The listing builds one solid part. Answer for the finished solid, in the listing's coordinates (mm). Face numbers are marked on the shaded views. A direction names the side the tool comes from. Give positions to 0.01 mm unless a question says otherwise; leave off trailing zeros. Write each loop counter-clockwise with the first axis right and the second up, starting at its lowest first coordinate (ties: lowest second). Pieces come first, ordered by that corner, then holes. Notation, with made-up numbers: (4.25, 28.25) - (48.25, 28.25) arc R21 cw to (48.25, 62.25) - close; hole circle Ø3 at (-23, 29.25). An arc over 180 degrees is marked (long way). Return JSON: item names as keys, results as strings.
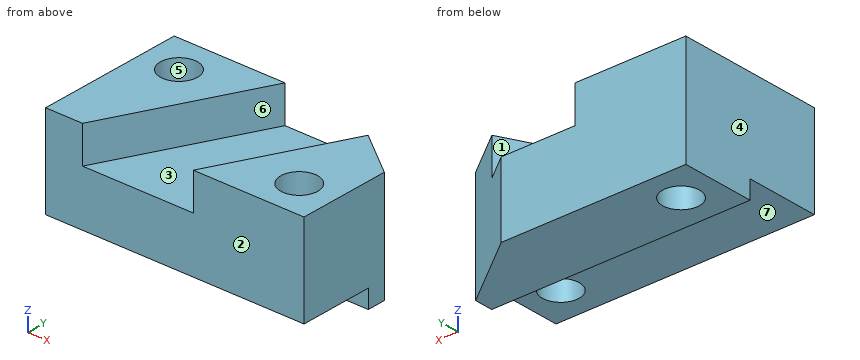
from build123d import *

# Parameters (mm, degrees)
SKETCH1_W               = 70
SKETCH1_H               = 30
BOSS_EXTRUDE1_DEPTH     = 40
CUT_EXTRUDE1_DEPTH      = 10
CUT_EXTRUDE2_DEPTH      = 1
CUT_EXTRUDE2_DEPTH_BACK = 31
SKETCH4_W               = 5
SKETCH4_H               = 20
CUT_EXTRUDE3_DEPTH      = 71
SKETCH5_R               = 5
CUT_EXTRUDE4_DEPTH      = 31
SKETCH6_R               = 5
CUT_EXTRUDE5_DEPTH      = 31


with BuildPart() as part:
    # Sketch1 → Boss-Extrude1 (new body)
    with BuildSketch(Plane(origin=(0, 0, 0), x_dir=(1, 0, 0), z_dir=(0, 1, 0))):
        with Locations((35, 15)):
            Rectangle(SKETCH1_W, SKETCH1_H)
    extrude(amount=BOSS_EXTRUDE1_DEPTH)

    # Sketch2 → Cut-Extrude1 (cut)
    with BuildSketch(Plane.XY):
        Polygon((30, 40), (10, 0), (40, 0), (60, 40), align=None)
    extrude(amount=-CUT_EXTRUDE1_DEPTH, mode=Mode.SUBTRACT)

    # Sketch3 → Cut-Extrude2 (cut, two sides)
    with BuildSketch(Plane(origin=(0, 0, -30), x_dir=(-1, 0, 0), z_dir=(0, 0, -1))) as cut_extrude2_sk:
        Polygon((-70, 40), (-70, 25), (-50, 40), align=None)
    extrude(amount=CUT_EXTRUDE2_DEPTH, mode=Mode.SUBTRACT)
    extrude(cut_extrude2_sk.sketch, amount=-CUT_EXTRUDE2_DEPTH_BACK, mode=Mode.SUBTRACT)

    # Sketch4 → Cut-Extrude3 (cut, through all)
    with BuildSketch(Plane(origin=(70, 0, 0), x_dir=(0, 0, -1), z_dir=(1, 0, 0))):
        with Locations((27.5, 10)):
            Rectangle(SKETCH4_W, SKETCH4_H)
    extrude(amount=-CUT_EXTRUDE3_DEPTH, mode=Mode.SUBTRACT)

    # Sketch5 → Cut-Extrude4 (cut, through all)
    with BuildSketch(Plane.XY):
        with Locations((60, 10)):
            Circle(SKETCH5_R)
    extrude(amount=-CUT_EXTRUDE4_DEPTH, mode=Mode.SUBTRACT)

    # Sketch6 → Cut-Extrude5 (cut, through all)
    with BuildSketch(Plane.XY):
        with Locations((10, 30)):
            Circle(SKETCH6_R)
    extrude(amount=-CUT_EXTRUDE5_DEPTH, mode=Mode.SUBTRACT)


solid = part.part
Item 1: Flat-ended cylindrical pins translate along their axes: P1, Ø8, axis at x = 51.5, y = 11, coming from the -Z side; P2, Ø2.5, axis at x = 32, z = -28, coming from the -Y side. Find the tip coordinate at first contact, or state that the pin passes through.
Answer below:
{"P1": "stops at z = -25", "P2": "stops at y = 20"}
Item 2: A cutting plane is placed at C-C on z = -22.5. Determine the outline of the cut face in (x, y).
Answer below:
{"outline": "(0, 0) - (70, 0) - (70, 25) - (50, 40) - (0, 40) - close; hole circle Ø10 at (10, 30); hole circle Ø10 at (60, 10)"}
Item 3: A cutting plane is placed at D-D on x = 18.5. Determine the outline of the cut face in (y, z).
Answer below:
{"outline": "(0, -25) - (20, -25) - (20, -30) - (40, -30) - (40, 0) - (17, 0) - (17, -10) - (0, -10) - close"}
Item 4: Consider L1, parallel to X at y = 7, z = -2.5; L2, parallel to X at y = 6, z = -1.25; L3, parallel to Y at x = 44, z = -26.75. Determine where each line is inside the solid, lowest interval first.
Answer below:
{"L1": "x = 0 to 13.5, 43.5 to 56, 64 to 70", "L2": "x = 0 to 13, 43 to 57, 63 to 70", "L3": "y = 20 to 40"}
Item 5: For the marked faces 1, 2 and 3, determine the directions among +Z, -Z, +X, -X, +Y, -Y from which every point of the face is accessible in a straight line to the end or side of a thin tool.
Answer below:
{"face 1": "+Z, +Y", "face 2": "+Z, -Z, +X, -X, -Y", "face 3": "+Z"}
Item 6: The mould has two halves that part along X. Classify the marked faces 4, 5, 6 and 7: +X half, -X half, draft (parallel to the pull), parting line (faces both ways), or undercut.
Answer below:
{"face 4": "-X half", "face 5": "undercut", "face 6": "undercut", "face 7": "draft"}
Item 7: A cutting plane is placed at B-B on x = 56. Determine the outline of the cut face in (y, z).
Answer below:
{"outline": "(0, -25) - (7, -25) - (7, 0) - (0, 0) - close; (13, -25) - (20, -25) - (20, -30) - (35.5, -30) - (35.5, -10) - (32, -10) - (32, 0) - (13, 0) - close"}
Item 8: A cutting plane is placed at A-A on y = 10. Determine the outline of the cut face in (x, z), then the cut area to 3 significant figures.
Answer below:
{"outline": "(0, -25) - (55, -25) - (55, 0) - (45, 0) - (45, -10) - (15, -10) - (15, 0) - (0, 0) - close; (65, -25) - (70, -25) - (70, 0) - (65, 0) - close", "area": "1,200 mm²"}
